Can you work these out from the model? Positions are in its coordinate system, mm. A direction names the side the tool comes from. Coordinates: 2 decimals unless noted, no trailing zeros. Loops run counter-clockwise (first coordinate to the right, second up) from the corner with the lowest first, then second, coordinate; pieces in that order, holes last. Notation, with made-up numbers: (-19, -33.5) -> (-10, -33.5) arc R20 ccw to (-10, -19.5) -> close; hole circle Ø3 at (-7.75, -33.5). An arc over 180 degrees is marked (long way). Put each result on its own line as item: value. Start each with the question number.
Item 1: If we section it at A-A on z = 1.1: Please give me the cut outline in (x, y).
Item 2: Will these pins go through, and if not, where does the flat tip stop? P1, Ø2.5, axis at y = 39, z = 2, coming from the +X side; P2, Ø1.5, axis at y = 27, z = 3.5, coming from the -X side; P3, Ø1.5, axis at x = -2, z = 2, coming from the -Y side.
Item 3: If we section it at B-B on x = 56.5: Please give me the cut outline in (y, z).
Item 4: For faces 1 (the flat face through (23, 170, 2)), 2 (the flat face through (128, 170, 2)), 3 (the flat face through (0, 30, 2)), which set-ups out of +Z, -Z, +X, -X, +Y, -Y let a thin tool reach every point of the face, with its end or its side?
Item 5: Please list where these lines run through material, in increasing order: L1, parallel to Y at x = 75, z = 2.15; L2, parallel to X at y = 155, z = 3.2; L3, parallel to Y at x = 72, z = 4.1. Write a range as from..to.
Item 6: If we section it at D-D on x = 38.5: Please give me the cut outline in (y, z), plus the area to 3 significant figures.
Item 7: We'd pull the mould along Y, two halves only. Please class faces 4 (the flat face through (105, 87, 2)), 5 (the flat face through (-2, 60, 2)), 6 (the flat face through (-3, 110, 2)): pulls with the +Y half, pulls with the -Y half, needs draft (parallel to the pull), parting line crosses it, or undercut.
Item 8: If we section it at C-C on y = 121.5: Please give me the cut outline in (x, z).
Autodesk Inventor part; units mm, degrees
ref_plane "YZ Plane" through (0, 0, 0) normal (1, 0, 0) x (0, 1, 0)
ref_plane "XZ Plane" through (0, 0, 0) normal (0, 1, 0) x (-1, 0, 0)
ref_plane "XY Plane" through (0, 0, 0) normal (0, 0, 1) x (1, 0, 0)
sketch "Sketch1" plane through (0, 0, 0) normal (0, 0, 1) x (1, 0, 0)
  line L0 (0, 0) -> (150, 0)
  line L1 (150, 0) -> (150, 170)
  line L2 (150, 170) -> (0, 170)
  line L3 (0, 170) -> (0, 0)
  line L4 (0, 60) -> (-5, 60)
  line L5 (-5, 60) -> (-5, 110)
  line L6 (-5, 110) -> (0, 110)
  line L7 (0, 110) -> (0, 60)
  line L8 (75, 0) -> (75, 170) construction
  line L9 (150, 60) -> (155, 60)
  line L10 (155, 60) -> (155, 110)
  line L11 (155, 110) -> (150, 110)
  line L12 (150, 110) -> (150, 60)
  line L13 (45, 85) -> (105, 85)
  line L14 (105, 85) -> (105, 90)
  line L15 (105, 90) -> (45, 90)
  line L16 (45, 90) -> (45, 85)
  line L17 (0, 85) -> (150, 85) construction
  line L18 (45, 170) -> (105, 170)
  line L19 (105, 170) -> (105, 175)
  line L20 (105, 175) -> (45, 175)
  line L21 (45, 175) -> (45, 170)
  point P0 (0, 110)
  point P1 (10, 0)
  point P2 (45, 87.5)
  dimension "d0" = 150
  dimension "d1" = 170
  dimension "d2" = 5
  dimension "d3" = 50
  dimension "d6" = 60
  dimension "d7" = 5
  dimension "d13" = 80
  dimension "d14" = 30
  dimension "d30" = 60
  dimension "d31" = 5
  dimension "d32" = 45
  dimension "d44" = 60
extrude "Extrusion1" add sketch "Sketch1" along normal blind 5
sketch "Sketch2" plane through (0, 0, 5) normal (0, 0, 1) x (1, 0, 0)
  line L0 (150, 170) -> (0, 170)
  line L1 (0, 0) -> (150, 0)
  line L2 (0, 170) -> (0, 110)
  line L3 (0, 60) -> (0, 0)
  point P0 (75, 20)
  dimension "d24" = 20
  dimension "d29" = 75
hole "Hole1" at (75, 20, 5) direction (0, 0, -1) diameter 3 end through all
sketch "Sketch3" plane through (0, 0, 5) normal (0, 0, 1) x (1, 0, 0)
  line L0 (105, 175) -> (45, 175)
  line L1 (45, 175) -> (45, 170)
  line L2 (0, 170) -> (0, 110)
  point P0 (0, 0)
  point P1 (75, 155)
  dimension "d40" = 20
  dimension "d45" = 75
hole "Hole2" at (75, 155, 5) direction (0, 0, -1) diameter 3 end through all
properties part number "back"
Solutions:
1. outline: (-5, 60) -> (0, 60) -> (0, 0) -> (150, 0) -> (150, 60) -> (155, 60) -> (155, 110) -> (150, 110) -> (150, 170) -> (105, 170) -> (105, 175) -> (45, 175) -> (45, 170) -> (0, 170) -> (0, 110) -> (-5, 110) -> close; hole (45, 85) -> (105, 85) -> (105, 90) -> (45, 90) -> close; hole circle Ø3 at (75, 20); hole circle Ø3 at (75, 155)
2. P1: x = 150
2. P2: x = 0
2. P3: y = 60
3. outline: (0, 0) -> (85, 0) -> (85, 5) -> (0, 5) -> close; (90, 0) -> (175, 0) -> (175, 5) -> (90, 5) -> close
4. face 1: +Z, -Z, -X, +Y
4. face 2: +Z, -Z, +X, +Y
4. face 3: +Z, -Z, -X, -Y
5. L1: 0..18.5, 21.5..85, 90..153.5, 156.5..175
5. L2: 0..73.5, 76.5..150
5. L3: 0..85, 90..175
6. outline: (0, 0) -> (170, 0) -> (170, 5) -> (0, 5) -> close
6. area: 850 mm^2
7. face 4: undercut
7. face 5: pulls with the -Y half
7. face 6: pulls with the +Y half
8. outline: (0, 0) -> (150, 0) -> (150, 5) -> (0, 5) -> close
